Read the model definition and answer for the solid it produces. Units are mm, in the model's axes. A direction names the side the tool comes from. Coordinates: 2 decimals unless noted, no trailing zeros. Answer as a JSON object with one key per item and string values. Group by question number.
1) Consider L1, parallel to Y at x = -2, z = 6.5; L2, parallel to Y at x = 0, z = 3.5; L3, parallel to X at y = 0, z = 7. Determine where each line is inside the solid, lowest interval first.
2) Given pin 1 (6 mm diameter, centred on y = 3, z = 3.5, fed in from -X); pin 2 (1.5 mm diameter, centred on y = -8, z = 7, fed in from -X); pin 3 (5 mm diameter, centred on x = -1, y = 0, fed in from -Z), each flat-ended and moving along its own axis, determine where each tip first touches the part or whether it passes through.
3) Determine the mould class of faces 1 (the cylindrical face through (-8, 0, 4)), 2 (the flat face through (0, 0, 12)), 3 (the flat face through (0, 3.4, 1)) for opening direction X: released by +X, released by -X, zero draft, split by the parting line, or undercut.
4) A tool of negligible diameter and unlimited length cuts with its end or side. For faces 4 (the flat face through (0, -3.4, 1)), 5 (the flat face through (4, 0, 0)), 6 (the cylindrical face through (2.77, 1.15, 7.25)), from which of +Z, -Z, +X, -X, +Y, -Y can it reach the whole face along a straight path? Write none if from no direction.
from build123d import *

# Parameters (mm, degrees)
F0_R     = 15.875
F1_DEPTH = 15
F3_R     = 3
F4_DEPTH = 12
F5_R     = 4
F6_DEPTH = 25


# Not quite as in the source:
# - a fillet or chamfer that OpenCascade refuses, or shapes differently, is made with other operations: its cross-section is extruded or revolved along the edge and cut away or added


with BuildPart() as f1:
    # F0 (on Top) → F1 (new body)
    with BuildSketch(Plane.XY):
        Circle(F0_R)
    extrude(amount=F1_DEPTH)

    # F2: fillet of radius 15.8 on 1 edges, made by hand

    # F2_s1 → F2_t2 (revolve, cut)
    with BuildSketch(Plane.XZ):
        with BuildLine():
            ThreePointArc((15.875, 0), (10.9810366905, 10.6516374375), (0.0952661619, 15))
            Line((0.0952661619, 15), (15.875, 15))
            Line((15.875, 15), (15.875, 0))
        make_face()
    revolve(axis=Axis((0, 0, 15), (0, 0, 1)), mode=Mode.SUBTRACT)

    # F3 (on face) → F4 (cut)
    with BuildSketch(Plane(origin=(0, 0, 0), x_dir=(1, 0, 0), z_dir=(0, 0, -1))):
        Circle(F3_R)
    extrude(amount=-F4_DEPTH, mode=Mode.SUBTRACT)

    # F5 (on Right) → F6 (cut)
    with BuildSketch(Plane.YZ):
        Circle(F5_R)
    extrude(amount=-F6_DEPTH, mode=Mode.SUBTRACT)


solid = f1.part
Worked answers:
{
 "1": {"L1": "y = -13.97 to -2.24, 2.24 to 13.97", "L2": "y = -15.3 to -3, 3 to 15.3", "L3": "x = -13.84 to -3, 3 to 13.84"},
 "2": {"pin 1": "stops at x = -15.33", "pin 2": "stops at x = -11.99", "pin 3": "stops at z = 3.24"},
 "3": {"face 1": "zero draft", "face 2": "undercut", "face 3": "released by -X"},
 "4": {"face 4": "-Z, -X", "face 5": "-Z, +X, -X, +Y, -Y", "face 6": "-Z"}
}
